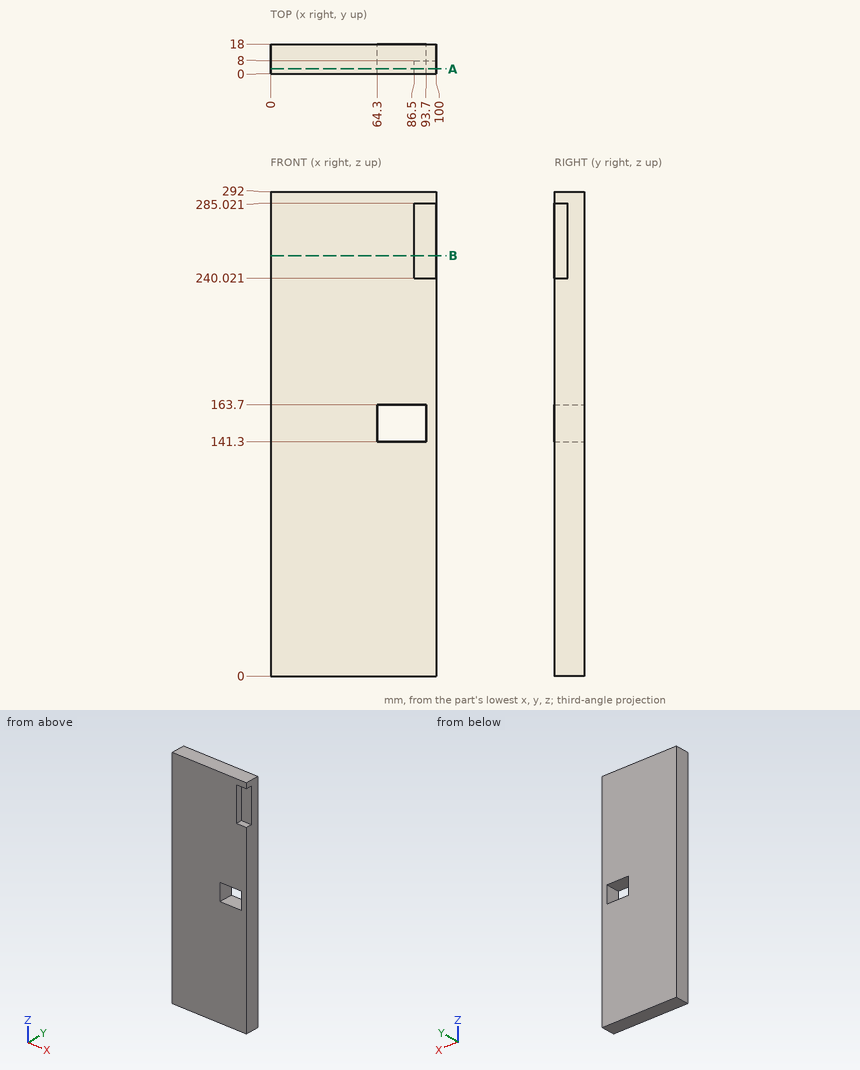
Design review of the part shown in the three views and the two pictorial views. Dimensions are in mm from the part's minimum x, y and z. Round coordinates to 2 decimals unless told otherwise and drop trailing zeros. Write each loop counter-clockwise with the first axis right and the second up, starting at its lowest first coordinate (ties: lowest second). Pieces come first, ordered by that corner, then holes. Notation, with made-up numbers: (85.5, -37.5) -> (92.5, -37.5) arc R14 cw to (92.5, -13.5) -> close; hole circle Ø4 at (22, -5). An arc over 180 degrees is marked (long way). Use one line per item in the form item = value.
1) Take a section at A-A, the plane y = 3. Write out the cut boundary in (x, z), and give its area (3 significant figures).
Found:
outline = (0, 0) -> (100, 0) -> (100, 240.02) -> (86.5, 240.02) -> (86.5, 285.02) -> (100, 285.02) -> (100, 292) -> (0, 292) -> close; hole (64.3, 141.3) -> (93.7, 141.3) -> (93.7, 163.7) -> (64.3, 163.7) -> close
area = 27,900 mm2
2) Clearance check with flat-ended pins moving along their axes: pin 1 (4 mm diameter, centred on y = 4.5, z = 268.5, fed in from +X); pin 2 (4 mm diameter, centred on x = 93, z = 253, fed in from -Y). State where each tip first meets the part, or that it passes through.
Found:
pin_1 = 86.5
pin_2 = 8
3) Take a section at B-B, the plane z = 253.5. Write out the cut boundary in (x, y), and give its area (3 significant figures).
Found:
outline = (0, 0) -> (86.5, 0) -> (86.5, 8) -> (100, 8) -> (100, 18) -> (0, 18) -> close
area = 1,690 mm2
4) To check wall thickness, follow L1, parallel to Z at x = 80, y = 14; L2, parallel to X at y = 11.75, z = 149. State the ranges of each line that lie inside material, in increasing order. Write a range as from..to.
Found:
L1 = 0..141.3, 163.7..292
L2 = 0..64.3, 93.7..100
